from build123d import *

# Parameters (mm, degrees)
F0_W     = 40
F0_H     = 22
F0_R     = 1.9
F0_R_2   = 2.4
F1_DEPTH = 5
F3_DEPTH = 2.3


with BuildPart() as f1:
    # F0 (on Front) → F1 (new body)
    with BuildSketch(Plane.XZ):
        with Locations((20, 11)):
            Rectangle(F0_W, F0_H)
        with Locations((7, 9.5)):
            Circle(F0_R, mode=Mode.SUBTRACT)
        with Locations((20, 9.5)):
            Circle(F0_R_2, mode=Mode.SUBTRACT)
        with Locations((33, 9.5)):
            Circle(F0_R, mode=Mode.SUBTRACT)
    extrude(amount=F1_DEPTH)

    # F2 (on face) → F3 (cut)
    with BuildSketch(Plane(origin=(0, 0, 0), x_dir=(-1, 0, 0), z_dir=(0, 1, 0))):
        Polygon((-14.5, 6.324574), (-14.5, 12.675426), (-20, 15.850853), (-25.5, 12.675426), (-25.5, 6.324574), (-20, 3.149147), align=None)
    extrude(amount=-F3_DEPTH, mode=Mode.SUBTRACT)


solid = f1.part
Work out the finished part from the listing and answer in its coordinate system (mm). A direction names the side the tool comes from. Give positions to 0.01 mm unless a question says otherwise; leave off trailing zeros. Write each loop counter-clockwise with the first axis right and the second up, starting at its lowest first coordinate (ties: lowest second). Pieces come first, ordered by that corner, then holes.
Q1. The part is cut by section C-C on x = 33. Give the vertices of the cut face in (y, z), and give its area (3 significant figures).
Answer:
outline: (-5, 0) - (0, 0) - (0, 7.6) - (-5, 7.6) - close; (-5, 11.4) - (0, 11.4) - (0, 22) - (-5, 22) - close
area: 91.0 mm2
Q2. Straight lines are drawn through the part: L1, parallel to Z at x = 33, y = -1.6; L2, parallel to X at y = -1.5, z = 11; L3, parallel to Z at x = 20, y = -3.5. For each, find the intervals that lie inside material, in ascending order.
Answer:
L1: z = 0 to 7.6, 11.4 to 22
L2: x = 0 to 5.83, 8.17 to 14.5, 25.5 to 31.83, 34.17 to 40
L3: z = 0 to 7.1, 11.9 to 22
Q3. For a pull along X with two mould halves and no side action, classify faces 3 (the face through (14.5, -1, 9)), 4 (the face through (40, -2, 11)), 5 (the face through (20, -5, 14)) as released by +X, released by -X, zero draft, split by the parting line, or undercut.
Answer:
face 3: undercut
face 4: released by +X
face 5: zero draft
Q4. The part is cut by section B-B on y = -1.5. Give the vertices of the cut face in (x, z).
Answer:
outline: (0, 0) - (40, 0) - (40, 22) - (0, 22) - close; hole circle Ø3.8 at (7, 9.5); hole (14.5, 6.32) - (20, 3.15) - (25.5, 6.32) - (25.5, 12.68) - (20, 15.85) - (14.5, 12.68) - close; hole circle Ø3.8 at (33, 9.5)
Q5. The part is cut by section A-A on z = 9.5. Give the vertices of the cut face in (x, y), and give its area (3 significant figures).
Answer:
outline: (0, -5) - (5.1, -5) - (5.1, 0) - (0, 0) - close; (8.9, -5) - (17.6, -5) - (17.6, -2.3) - (14.5, -2.3) - (14.5, 0) - (8.9, 0) - close; (22.4, -5) - (31.1, -5) - (31.1, 0) - (25.5, 0) - (25.5, -2.3) - (22.4, -2.3) - close; (34.9, -5) - (40, -5) - (40, 0) - (34.9, 0) - close
area: 124 mm2
Q6. A tool of negligible diameter and unlimited length cuts with its end or side. For faces 1 (the face through (5.492, -2.465, 8.344)), 2 (the face through (17.21, -1.13, 14.24)), from which of +Z, -Z, +X, -X, +Y, -Y can it reach the whole face along a straight path? Write none if from no direction.
Answer:
face 1: +Y, -Y
face 2: +Y
Q7. The part is cut by section D-D on z = 5. Give the vertices of the cut face in (x, y).
Answer:
outline: (0, -5) - (40, -5) - (40, 0) - (23.21, 0) - (23.21, -2.3) - (16.79, -2.3) - (16.79, 0) - (0, 0) - close
